```python
from build123d import *

# Parameters (mm, degrees)
SKETCH1_R           = 1.65
BOSS_EXTRUDE1_DEPTH = 10
SKETCH2_R           = 2
CUT_EXTRUDE1_DEPTH  = 18.495331881
FILLET1_R           = 1


with BuildPart() as part:
    # Sketch1 → Boss-Extrude1 (new body)
    with BuildSketch(Plane.XY):
        with BuildLine():
            Line((12.688854384, 4.179140788), (-42.311145616, 4.179140788))
            ThreePointArc((-42.311145616, 4.179140788), (-46.311145616, 0.179140788), (-42.311145616, -3.820859212))
            Line((-42.311145616, -3.820859212), (15.288854384, -3.820859212))
            Line((15.288854384, -3.820859212), (29.430990008, 10.321276412))
            Line((29.430990008, 10.321276412), (24.130990008, 15.621276412))
            Line((24.130990008, 15.621276412), (12.688854384, 4.179140788))
        make_face()
        with Locations((-34.711145616, 0.179140788)):
            Circle(SKETCH1_R, mode=Mode.SUBTRACT)
        with Locations((-42.311145616, 0.179140788)):
            Circle(SKETCH1_R, mode=Mode.SUBTRACT)
    extrude(amount=BOSS_EXTRUDE1_DEPTH)

    # Sketch2 → Cut-Extrude1 (cut, through all)
    with BuildSketch(Plane(origin=(4.254856798, -4.254856798, 0), x_dir=(0, 0, 1), z_dir=(-0.707106781, 0.707106781, 0))):
        with Locations((5, 20.018285462)):
            Circle(SKETCH2_R)
    extrude(amount=-CUT_EXTRUDE1_DEPTH, mode=Mode.SUBTRACT)

    # Fillet1
    fillet1_edges = [part.edges().sort_by_distance(p)[0] for p in [
        (26.780990008, 12.971276412, 0),
        (26.780990008, 12.971276412, 10),
    ]]
    fillet(fillet1_edges, radius=FILLET1_R)


solid = part.part
```
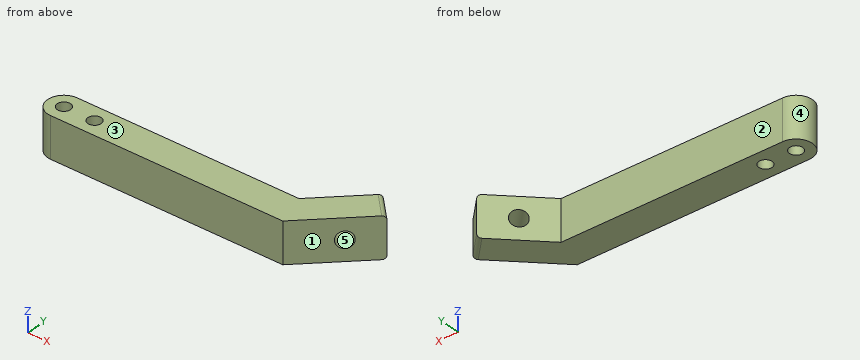
Input: part model. Units: mm. Frame: model coordinates. Face numbers are marked on the shaded views. A direction names the side the tool comes from. Give positions to 0.01 mm unless a question says otherwise; leave off trailing zeros. Order: outer loops, then holes, each group sorted by start corner. A loop starts at its lowest first (then second) coordinate and runs counter-clockwise, first axis right, second up. Notation, with made-up numbers: M -32.75,71.5 L 11.25,71.5 A34 cw 11.25,108.5 Z; hole C 11,24.5 d6. An arc over 180 degrees is marked long. Return JSON: item names as keys, results as strings.
Item 1: Cut plane B-B (y = -0.75). Return loops of the section in (x, z), then the cut area to 3 significant figures.
Solutions:
{"outline": "M -46.2,0 L -43.67,0 L -43.67,10 L -46.2,10 Z; M -40.95,0 L -36.07,0 L -36.07,10 L -40.95,10 Z; M -33.35,0 L 18.36,0 L 18.36,10 L -33.35,10 Z", "area": "591 mm^2"}
Item 2: Access query for the marked faces 1 and 2. Directions: +Z, -Z, +X, -X, +Y, -Y. A direction counts if a zero-diameter tool reaches every point of the face in a straight line with its end or side. Return the directions, or none.
Solutions:
{"face 1": "+Z, -Z, +X, -Y", "face 2": "+Z, -Z, -X, +Y"}
Item 3: Cut plane D-D (x = 14). Return loops of the section in (y, z).
Solutions:
{"outline": "M -3.82,0 L 5.49,0 L 5.49,10 L -3.82,10 Z"}
Item 4: First-contact query: P1, Ø2, axis at y = 10, z = 3.5, coming from the -X side; P2, Ø6, axis at x = -34.5, z = 4.5, coming from the +Y side; P3, Ø3, axis at y = 4.5, z = 3.5, coming from the -X side. Flat tips, straight axial feed; report the tip coordinate or a pass-through.
Solutions:
{"P1": "x = 17.51", "P2": "y = 4.18", "P3": "x = -45.15"}
Item 5: Cut plane C-C (x = -28.5). Return loops of the section in (y, z), then the cut area to 3 significant figures.
Solutions:
{"outline": "M -3.82,0 L 4.18,0 L 4.18,10 L -3.82,10 Z", "area": "80.0 mm^2"}
Item 6: Cut plane A-A (z = 5). Return loops of the section in (x, y).
Solutions:
{"outline": "M -42.31,-3.82 L 15.29,-3.82 L 22.3,3.19 L 17,8.49 L 12.69,4.18 L -42.31,4.18 A4 ccw Z; M 19.82,11.31 L 25.12,6.01 L 29.43,10.32 L 24.13,15.62 Z; hole C -42.31,0.18 d3.3; hole C -34.71,0.18 d3.3"}
Item 7: Ray query, probe 1 along Y at (x, z) = (-34.5, 1.75); probe 2 along X at (y, z) = (1.25, 2); probe 3 along Y at (x, z) = (-13, 4). Return the intervals inside material, ascending.
Solutions:
{"probe 1": "-3.82 to -1.46, 1.82 to 4.18", "probe 2": "-46.17 to -43.57, -41.06 to -35.97, -33.46 to 20.36", "probe 3": "-3.82 to 4.18"}
Item 8: Pull-direction query (Y, two-part tool) for the marked faces 3, 4 and 5; classes: +Y half, -Y half, draft (parallel to the pull), parting line (faces both ways), or undercut.
Solutions:
{"face 3": "draft", "face 4": "parting line", "face 5": "undercut"}
